Source: three-view drawing plus pictorial views. Frame: mm from the lowest corner of the part. Give positions to 0.01 mm unless a question says otherwise; leave off trailing zeros. Order: outer loops, then holes, each group sorted by start corner. A loop starts at its lowest first (then second) coordinate and runs counter-clockwise, first axis right, second up.
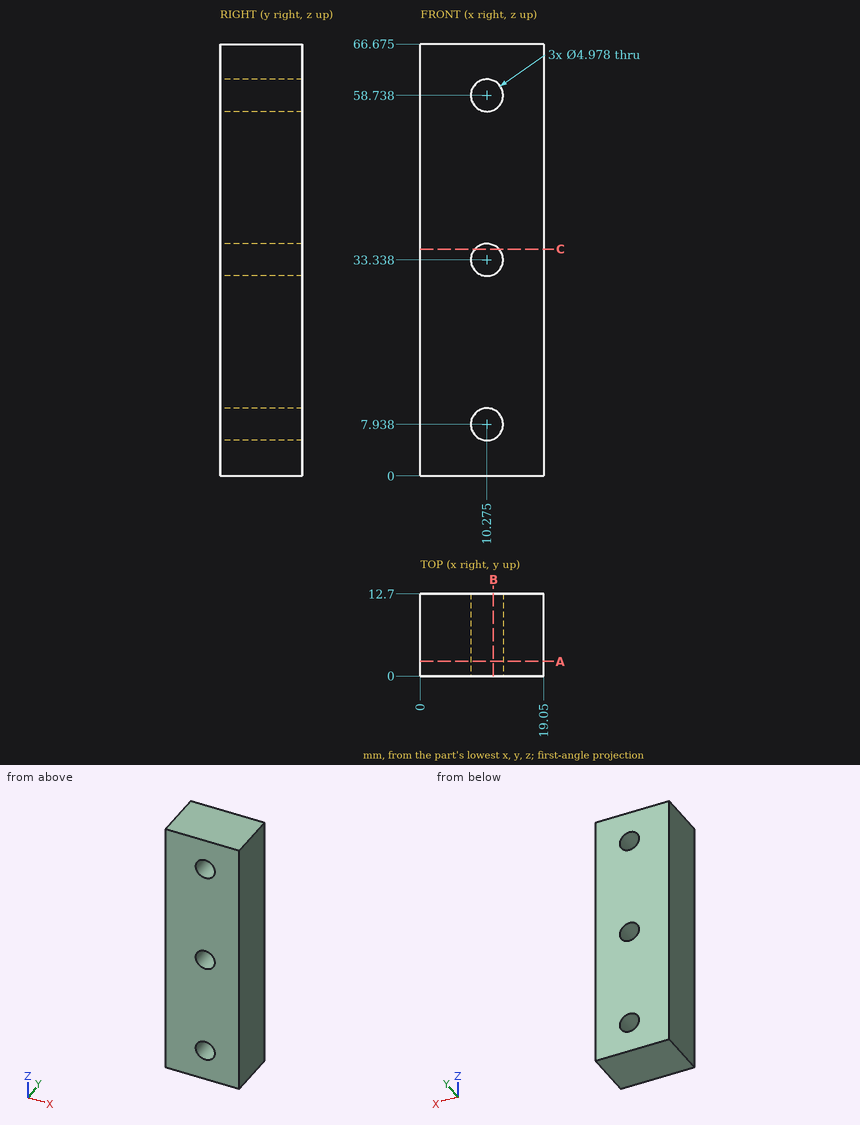
(1) Pin query (flat end, axial travel): pin 1 Ø4 at (x, z) = (10.27, 7.94) entering from -Y. Return the tip coordinate at first contact, or that it passes through.
(2) Section C-C, the plane z = 35. Return loops of the section in (x, y), plus the area to 3 significant figures.
(3) Section A-A, the plane y = 2.25. Count the separate pieces of the cut face and the enclosed holes in it, plus the area to 3 significant figures.
(4) Section B-B, the plane x = 11.25. Return loops of the section in (y, z) (1 decimal).
(5) Line query: line 1 along Z through (x, y) = (9.5, 2.5) (1 decimal); line 2 along Z through (x, y) = (12, 2) (1 decimal). Output: solid intervals per line, ascending.
Checks:
1. pin 1: passes through
2. outline: (0, 0) - (8.42, 0) - (8.42, 12.7) - (0, 12.7) - close; (12.13, 0) - (19.05, 0) - (19.05, 12.7) - (12.13, 12.7) - close
2. area: 195 mm2
3. separate pieces: 1
3. enclosed holes: 3
3. area: 1,210 mm2
4. outline: (0, 0) - (12.7, 0) - (12.7, 5.6) - (0, 5.6) - close; (0, 10.2) - (12.7, 10.2) - (12.7, 31) - (0, 31) - close; (0, 35.6) - (12.7, 35.6) - (12.7, 56.4) - (0, 56.4) - close; (0, 61) - (12.7, 61) - (12.7, 66.7) - (0, 66.7) - close
5. line 1: z = 0 to 5.6, 10.3 to 31, 35.7 to 56.4, 61.1 to 66.7
5. line 2: z = 0 to 6.1, 9.7 to 31.5, 35.1 to 56.9, 60.5 to 66.7
